Verification items for this drawing (mm, ordinates from the low corner). A direction names the side the tool comes from. Coordinates: 2 decimals unless noted, no trailing zeros. Loops run counter-clockwise (first coordinate to the right, second up) from the corner with the lowest first, then second, coordinate; pieces in that order, holes last. Notation, with made-up numbers: M 85,28 L 127,28 A27 ccw 127,61 Z; hole C -12,32 d6. An arc over 180 degrees is marked long. Return JSON: item names as keys, results as strings.
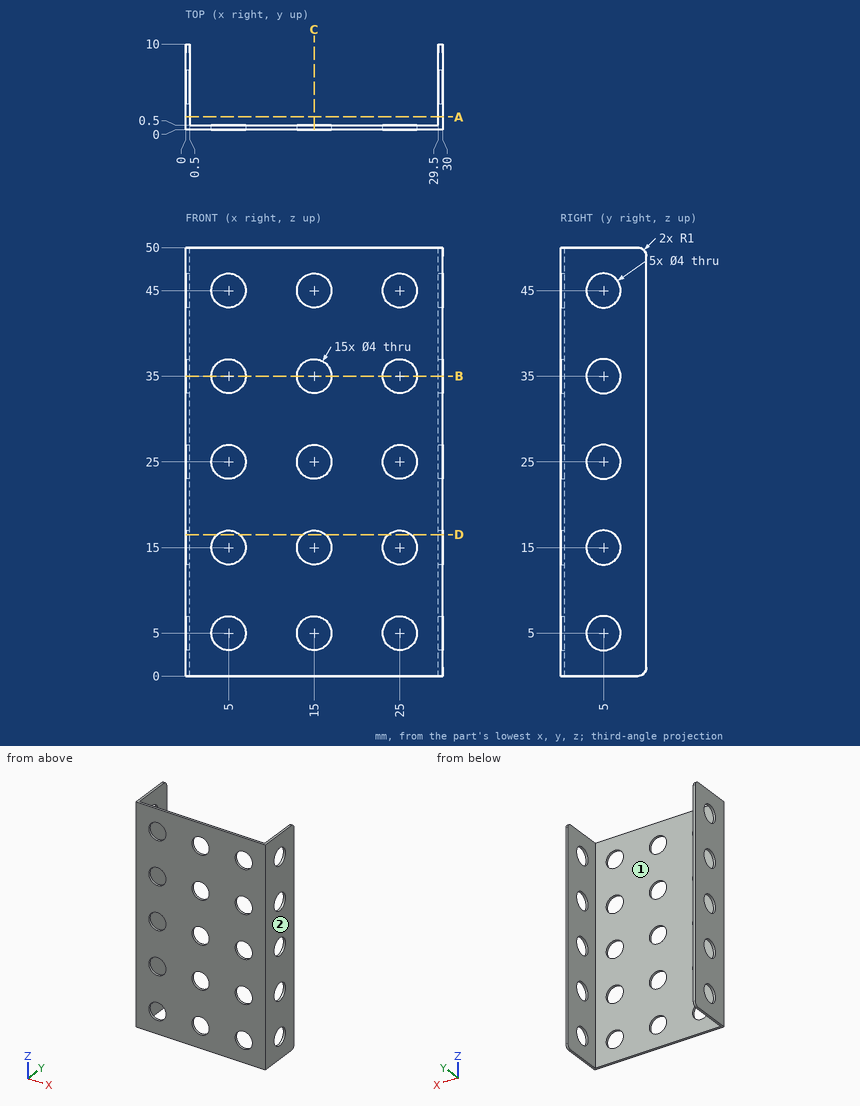
1) Section check B-B on z = 35. Record the cut outline in (x, y).
Answers:
{"outline": "M 0,0 L 3,0 L 3,0.5 L 0.5,0.5 L 0.5,3 L 0,3 Z; M 0,7 L 0.5,7 L 0.5,10 L 0,10 Z; M 7,0 L 13,0 L 13,0.5 L 7,0.5 Z; M 17,0 L 23,0 L 23,0.5 L 17,0.5 Z; M 27,0 L 30,0 L 30,3 L 29.5,3 L 29.5,0.5 L 27,0.5 Z; M 29.5,7 L 30,7 L 30,10 L 29.5,10 Z"}
2) Scan lines: line 1 along X through (y, z) = (0.2, 35); line 2 along Z through (x, y) = (5, 0.2); line 3 along X through (y, z) = (2.5, 33). Record each from-to range of solid material in increasing order. Write a range as [from, to].
Answers:
{"line 1": "[0, 3], [7, 13], [17, 23], [27, 30]", "line 2": "[0, 3], [7, 13], [17, 23], [27, 33], [37, 43], [47, 50]", "line 3": "[0, 0.5], [29.5, 30]"}
3) Section check D-D on z = 16.5. Record the cut outline in (x, y), then the cut area to 3 significant figures.
Answers:
{"outline": "M 0,0 L 3.68,0 L 3.68,0.5 L 0.5,0.5 L 0.5,3.68 L 0,3.68 Z; M 0,6.32 L 0.5,6.32 L 0.5,10 L 0,10 Z; M 6.32,0 L 13.68,0 L 13.68,0.5 L 6.32,0.5 Z; M 16.32,0 L 23.68,0 L 23.68,0.5 L 16.32,0.5 Z; M 26.32,0 L 30,0 L 30,3.68 L 29.5,3.68 L 29.5,0.5 L 26.32,0.5 Z; M 29.5,6.32 L 30,6.32 L 30,10 L 29.5,10 Z", "area": "17.9 mm²"}
4) Go/stop test with flat-tipped pins: pin 1 Ø5 at (y, z) = (5, 5) entering from +X; pin 2 Ø1.5 at (x, z) = (23, 37.5) entering from +Y. Record where each tip stops, or that it passes through.
Answers:
{"pin 1": "x = 30", "pin 2": "y = 0.5"}
5) Section check A-A on y = 1.5. Record the cut outline in (x, z), then the cut area to 3 significant figures.
Answers:
{"outline": "M 0,0 L 0.5,0 L 0.5,50 L 0,50 Z; M 29.5,0 L 30,0 L 30,50 L 29.5,50 Z", "area": "50.0 mm²"}
6) Set-up check for the marked faces 1 and 2: record each of +Z, -Z, +X, -X, +Y, -Y from which the full face is reachable in a straight line by a thin tool's end or side.
Answers:
{"face 1": "+Z, -Z, +Y", "face 2": "+Z, -Z, +X, +Y, -Y"}
7) Section check C-C on x = 15. Record the cut outline in (y, z).
Answers:
{"outline": "M 0,0 L 0.5,0 L 0.5,3 L 0,3 Z; M 0,7 L 0.5,7 L 0.5,13 L 0,13 Z; M 0,17 L 0.5,17 L 0.5,23 L 0,23 Z; M 0,27 L 0.5,27 L 0.5,33 L 0,33 Z; M 0,37 L 0.5,37 L 0.5,43 L 0,43 Z; M 0,47 L 0.5,47 L 0.5,50 L 0,50 Z"}
